Input: dimensioned drawing with shaded views. Units: mm. Origin: part minimum x, y, z. Give positions to 0.01 mm unless a question says otherwise; leave off trailing zeros. Write each loop counter-clockwise with the first axis right and the second up, starting at its lowest first coordinate (ties: lowest second). Pieces come first, ordered by that corner, then holes. Notation, with made-up numbers: (84.5, 55.25) -> (129.5, 55.25) arc R21 ccw to (129.5, 62.25) -> close; hole circle Ø10 at (-29, 64). An arc over 180 degrees is marked (long way). Answer as a JSON object with one key per item and string values.
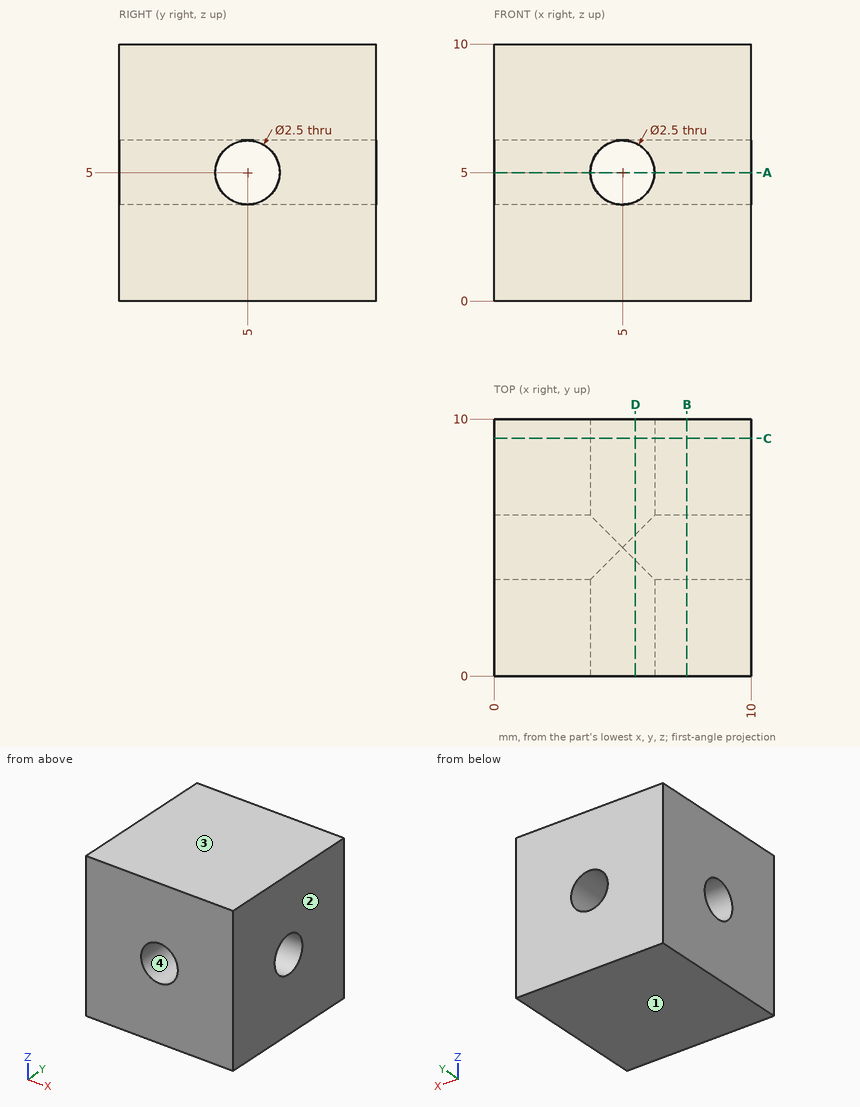
Q1. Cut plane B-B (x = 7.5). Return the cut outline in (y, z).
Values:
{"outline": "(0, 0) -> (10, 0) -> (10, 10) -> (0, 10) -> close; hole circle Ø2.5 at (5, 5)"}
Q2. Material intervals for L1, parallel to Y at x = 1.1, z = 5; L2, parallel to Z at x = 2.25, y = 4.25, sorted ascending. Write a range as from..to.
Values:
{"L1": "0..3.75, 6.25..10", "L2": "0..4, 6..10"}
Q3. Mould query, pull axis Z, two halves, no side actions, for the marked faces 1, 2, 3 and 4. Classes: pulls with the +Z half, pulls with the -Z half, needs draft (parallel to the pull), parting line crosses it, or undercut.
Values:
{"face 1": "pulls with the -Z half", "face 2": "needs draft", "face 3": "pulls with the +Z half", "face 4": "undercut"}
Q4. Cut plane D-D (x = 5.5). Return the cut outline in (y, z).
Values:
{"outline": "(0, 0) -> (10, 0) -> (10, 3.85) -> (5.5, 3.85) arc R1.25 cw to (4.5, 3.85) -> (0, 3.85) -> close; (0, 6.15) -> (4.5, 6.15) arc R1.25 cw to (5.5, 6.15) -> (10, 6.15) -> (10, 10) -> (0, 10) -> close"}
Q5. Cut plane A-A (z = 5). Return the cut outline in (x, y), and give its area (4 significant figures).
Values:
{"outline": "(0, 0) -> (3.75, 0) -> (3.75, 3.75) -> (0, 3.75) -> close; (0, 6.25) -> (3.75, 6.25) -> (3.75, 10) -> (0, 10) -> close; (6.25, 0) -> (10, 0) -> (10, 3.75) -> (6.25, 3.75) -> close; (6.25, 6.25) -> (10, 6.25) -> (10, 10) -> (6.25, 10) -> close", "area": "56.25 mm²"}
